Could you check a few things on this model? Use its own coordinates, in mm. A direction names the side the tool comes from. Coordinates: 2 decimals unless noted, no trailing zeros. Write each loop counter-clockwise with the first axis right and the second up, starting at its lowest first coordinate (ties: lowest second). Pieces come first, ordered by that corner, then holes. Notation, with made-up numbers: M 44,-4.75 L 72,-4.75 A33 cw 72,26.25 Z; hole C 42,78 d6. An arc over 180 degrees is marked long. Answer as CSV lines item,"result". Start each with the question number.
Item 1: On a 3-axis mill with a long thin cutter (end or side, diameter ignored), from which of +Z, -Z, +X, -X, +Y, -Y can I reach the whole of each face in a straight line? I mean faces 1 (the flat face through (-12.7, -9, -16)), 2 (the flat face through (0, 0, 15)), 3 (the cylindrical face through (-26.585, -15.831, 22.32)). Say none if no direction works.
Item 2: I'm going to push flat-ended pins straight in: P1, Ø10, axis at x = 12.5, z = 5.5, coming from the +Y side; P2, Ø5, axis at x = 23.57, z = 23.57, coming from the -Y side; P3, Ø6, axis at x = -1, y = -10, coming from the -Z side; P4, Ø6, axis at x = -23.57, z = -23.57, coming from the -Y side. Where does each tip first touch, or does it pass through?
Item 3: Suppose I cut it at D-D, the plane x = -9.5. Write out the boundary of the cut face in (y, z), and give its area (3 significant figures).
Item 4: If I drill on line 1 along X through (y, z) = (-15.75, 23.57); line 2 along X through (y, z) = (-14.25, -23.57); line 3 along X through (y, z) = (-13.25, -9), over which ranges is the centre line in solid material (lowest first)? Write a range as [from, to].
Item 5: Suppose I cut it at C-C, the plane y = -7.75. Write out the boundary of the cut face in (x, z), and give its area (3 significant figures).
Item 6: Suppose I cut it at A-A, the plane y = -14.5. Write out the boundary of the cut face in (x, z).
Item 7: Suppose I cut it at B-B, the plane z = -16. Write out the boundary of the cut face in (x, y), and give its area (3 significant figures).
```python
from build123d import *

# Parameters (mm, degrees)
F1_DEPTH = 19.05
F3_D     = 6.5278
F3_DEPTH = 6.35
F3_TIP   = 1.9611489744
F5_D     = 6.5278


with BuildPart() as f1:
    # F0 (on Front) → F1 (new body)
    with BuildSketch(Plane.XZ):
        with BuildLine():
            Line((31.75, 31.75), (-31.75, 31.75))
            Line((-31.75, 31.75), (-31.75, -31.75))
            Line((-31.75, -31.75), (-12.7, -31.75))
            Line((-12.7, -31.75), (-12.7, 0))
            ThreePointArc((-12.7, 0), (0, 12.7), (12.7, 0))
            Line((12.7, 0), (12.7, -31.75))
            Line((12.7, -31.75), (31.75, -31.75))
            Line((31.75, -31.75), (31.75, 31.75))
        make_face()
    extrude(amount=F1_DEPTH)

    # F3
    with Locations(Plane.XZ.offset(19.05)):
        with Locations((-23.57, 23.57), (-23.57, -23.57), (23.57, -23.57), (23.57, 23.57)):
            Hole(F3_D / 2, depth=F3_DEPTH)
            with Locations((0, 0, -(F3_DEPTH + F3_TIP / 2))):  # 118° drill point
                Cone(0, F3_D / 2, F3_TIP, mode=Mode.SUBTRACT)

    # F5 (through all)
    with Locations(Plane.XZ.offset(19.05)):
        with Locations((-21.43125, 0), (21.43125, 0)):
            Hole(F5_D / 2)


solid = f1.part
```
Ans:
1,face 1,"-Z, +Y, -Y"
1,face 2,"+Z, -Z, +X, -X, +Y"
1,face 3,"-Y"
2,P1,"stops at y = 0"
2,P2,"stops at y = -12.24"
2,P3,"stops at z = 12.05"
2,P4,"stops at y = -12.54"
3,outline,"M -19.05,8.43 L 0,8.43 L 0,31.75 L -19.05,31.75 Z"
3,area,"444 mm^2"
4,line 1,"x = [-31.75, -26.83], [-20.31, 20.31], [26.83, 31.75]"
4,line 2,"x = [-31.75, -26.83], [-20.31, -12.7], [12.7, 20.31], [26.83, 31.75]"
4,line 3,"x = [-31.75, -12.7], [12.7, 31.75]"
5,outline,"M -31.75,-31.75 L -12.7,-31.75 L -12.7,0 A12.7 cw 12.7,0 L 12.7,-31.75 L 31.75,-31.75 L 31.75,31.75 L -31.75,31.75 Z; hole C -21.43,0 d6.53; hole C 21.43,0 d6.53"
5,area,"2,910 mm^2"
6,outline,"M -31.75,-31.75 L -12.7,-31.75 L -12.7,0 A12.7 cw 12.7,0 L 12.7,-31.75 L 31.75,-31.75 L 31.75,31.75 L -31.75,31.75 Z; hole C -23.57,-23.57 d6.53; hole C -23.57,23.57 d6.53; hole C -21.43,0 d6.53; hole C 21.43,0 d6.53; hole C 23.57,-23.57 d6.53; hole C 23.57,23.57 d6.53"
7,outline,"M -31.75,-19.05 L -12.7,-19.05 L -12.7,0 L -31.75,0 Z; M 12.7,-19.05 L 31.75,-19.05 L 31.75,0 L 12.7,0 Z"
7,area,"726 mm^2"
